Job drawing, mm, ordinate dimensions from the low corner. One solid piece. A direction names the side the tool comes from. Round coordinates to 2 decimals unless told otherwise and drop trailing zeros. Write each loop counter-clockwise with the first axis right and the second up, starting at its lowest first coordinate (ties: lowest second). Pieces come first, ordered by that corner, then holes. Notation, with made-up numbers: (25.25, -12) -> (35.25, -12) arc R27 cw to (35.25, 15) -> close; hole circle Ø1 at (-5, 3.25). An arc over 180 degrees is marked (long way). Use CSV: the item, a comma, the result in double quotes. Start each with the question number.
(1) Which spindle directions (+Z, -Z, +X, -X, +Y, -Y) get a long thin tool onto all of the face, cutting with end or side? Do the marked faces 1, 2 and 3. Say none if no direction does.
(2) Probe line 1 (Y direction, x = 14.25, z = 2.5); line 2 (X direction, y = 3.45, z = 3.5); line 3 (Y direction, x = 3.75, z = 21). List the from-to ranges inside material, lowest first. Write a range as [from, to].
(3) Saw through at A-A (y = 2.5). Give the cut face in (x, z), plus the area to 3 significant figures.
(4) Saw through at C-C (y = 4.5). Give the cut face in (x, z), plus the area to 3 significant figures.
(5) Drop flat-ended pins along their axis: pin 1 (8 mm diameter, centred on x = 16, z = 15, fed in from +Y); pin 2 (1.3 mm diameter, centred on y = 3.5, z = 1.5, fed in from +X); pin 3 (5 mm diameter, centred on x = 8.5, z = 18.5, fed in from -Y). Give the stop position or say it passes through.
(6) Saw through at B-B (z = 2.5). Give the cut face in (x, y).
(7) Saw through at D-D (x = 2.25). Give the cut face in (y, z).
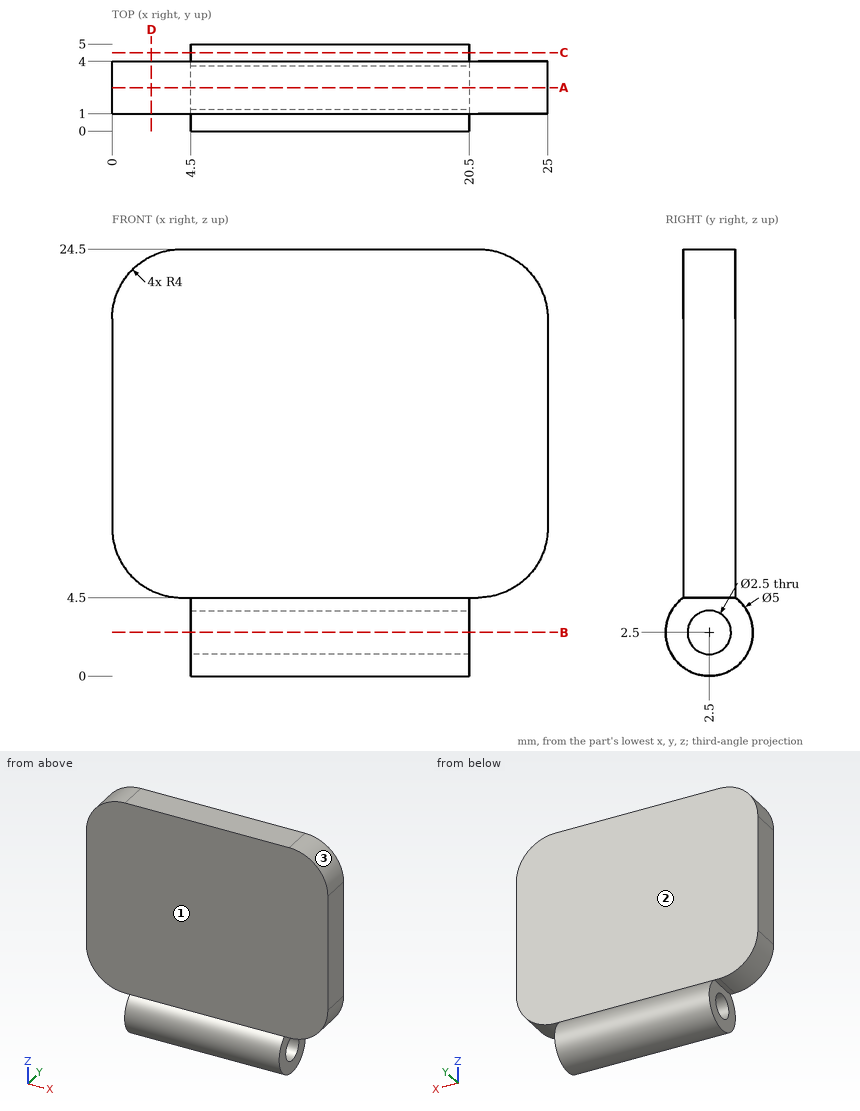
Answers:
1,face 1,"+Z, +X, -X, -Y"
1,face 2,"+Z, +X, -X, +Y"
1,face 3,"+Z, +X, +Y, -Y"
2,line 1,"y = [0, 1.25], [3.75, 5]"
2,line 2,"x = [4.5, 20.5]"
2,line 3,"y = [1, 4]"
3,outline,"(0, 8.5) arc R4 ccw to (4, 4.5) -> (4.5, 4.5) -> (4.5, 3.75) -> (20.5, 3.75) -> (20.5, 4.5) -> (21, 4.5) arc R4 ccw to (25, 8.5) -> (25, 20.5) arc R4 ccw to (21, 24.5) -> (4, 24.5) arc R4 ccw to (0, 20.5) -> close; (4.5, 0) -> (20.5, 0) -> (20.5, 1.25) -> (4.5, 1.25) -> close"
3,area,"518 mm²"
4,outline,"(4.5, 1) -> (20.5, 1) -> (20.5, 4) -> (4.5, 4) -> close"
4,area,"48.0 mm²"
5,pin 1,"stops at y = 4"
5,pin 2,"stops at x = 20.5"
5,pin 3,"stops at y = 1"
6,outline,"(4.5, 0) -> (20.5, 0) -> (20.5, 1.25) -> (4.5, 1.25) -> close; (4.5, 3.75) -> (20.5, 3.75) -> (20.5, 5) -> (4.5, 5) -> close"
7,outline,"(1, 4.9) -> (4, 4.9) -> (4, 24.1) -> (1, 24.1) -> close"
